from build123d import *

# Parameters (mm, degrees)
F0_R     = 3.5
F0_R_2   = 2.15
F0_R_3   = 1.65
F1_DEPTH = 1
F2_R     = 2.15
F2_R_2   = 1.65
F3_DEPTH = 2
F4_R     = 2.75
F4_R_2   = 2.15
F4_R_3   = 1.65
F5_DEPTH = 1
F6_SIZE  = 0.59999


# Not quite as in the source:
# - a fillet or chamfer is up to 0.001 mm smaller than in the source, because OpenCascade refuses the exact size


with BuildPart() as f1:
    # F0 (on Top) → F1 (new body)
    with BuildSketch(Plane.XY):
        Circle(F0_R)
        Circle(F0_R_2, mode=Mode.SUBTRACT)
        Circle(F0_R_2)
        Circle(F0_R_3, mode=Mode.SUBTRACT)
    extrude(amount=F1_DEPTH)

    # F2 (on face) → F3 (join)
    with BuildSketch(Plane.XY.offset(1)):
        Circle(F2_R)
        Circle(F2_R_2, mode=Mode.SUBTRACT)
    extrude(amount=F3_DEPTH)

    # F4 (on face) → F5 (join)
    with BuildSketch(Plane.XY.offset(3)):
        Circle(F4_R)
        Circle(F4_R_2, mode=Mode.SUBTRACT)
        Circle(F4_R_2)
        Circle(F4_R_3, mode=Mode.SUBTRACT)
    extrude(amount=F5_DEPTH)

    # F6 (size 0.6 in the source; OpenCascade refuses exactly that, so slightly less here)
    f6_edges = [f1.edges().sort_by_distance(p)[0] for p in [
        (-2.75, 0, 3),
    ]]
    chamfer(f6_edges, length=F6_SIZE)


solid = f1.part
Geometry check sheet. Reference: the model listing, model coordinates, mm. A direction names the side the tool comes from. Give positions to 0.01 mm unless a question says otherwise; leave off trailing zeros. Loops run counter-clockwise (first coordinate to the right, second up) from the corner with the lowest first, then second, coordinate; pieces in that order, holes last. Notation, with made-up numbers: (82, 59) -> (111, 59) arc R32 ccw to (111, 91) -> close; hole circle Ø10 at (-38.5, -27). An arc over 180 degrees is marked (long way). Answer in a Markdown table with one row per item. Add a question column.
1) Gauge pin test, flat ends, axial feed: P1, Ø4, axis at x = 1.5, y = 2, coming from the -Z side; P2, Ø2, axis at x = 0, y = 0, coming from the -Z side. Record the tip position at first contact, or that the pin passes through.
2) Cross-section at C-C on z = 0.75. Record the boundary of the cut face in (x, y), and give its area (3 significant figures).
3) Material ranges on probe 1 along Y at (x, z) = (0, 2.5); probe 2 along Y at (x, z) = (-0.75, 2.4); probe 3 along X at (y, z) = (-1, 3.55), recorded low to high. Write a range as from..to.
4) Draft check along Z on faces 4 (the face through (-2, -2, 1)), 5 (the face through (1, -2, 0)), 6 (the face through (2, 0, 4)). Enter one of: pulls with the +Z half, pulls with the -Z half, needs draft (parallel to the pull), parting line crosses it, or undercut.
5) Cross-section at D-D on z = 3.2. Record the boundary of the cut face in (x, y).
6) Set-up check for faces 1 (the face through (3.233, -1.341, 0.493)), 2 (the face through (-2.15, 0.09, 1.99)), 3 (the face through (-0.596, -2.685, 3.797)): record each of +Z, -Z, +X, -X, +Y, -Y from which the full face is reachable in a straight line by a thin tool's end or side.
Outcome:
| question | item | result |
|---|---|---|
| 1 | P1 | stops at z = 0 |
| 1 | P2 | passes through |
| 2 | outline | circle Ø7 at (0, 0); hole circle Ø3.3 at (0, 0) |
| 2 | area | 29.9 mm^2 |
| 3 | probe 1 | y = -2.15..-1.65, 1.65..2.15 |
| 3 | probe 2 | y = -2.01..-1.47, 1.47..2.01 |
| 3 | probe 3 | x = -2.51..-1.31, 1.31..2.51 |
| 4 | face 4 | undercut |
| 4 | face 5 | pulls with the -Z half |
| 4 | face 6 | pulls with the +Z half |
| 5 | outline | circle Ø4.7 at (0, 0); hole circle Ø3.3 at (0, 0) |
| 6 | face 1 | +Z, -Z |
| 6 | face 2 | none |
| 6 | face 3 | +Z |
